Design review of the part shown in the three views and the two pictorial views. Dimensions are in mm from the part's minimum x, y and z. A direction names the side the tool comes from. Give positions to 0.01 mm unless a question says otherwise; leave off trailing zeros. Loops run counter-clockwise (first coordinate to the right, second up) from the corner with the lowest first, then second, coordinate; pieces in that order, holes last.
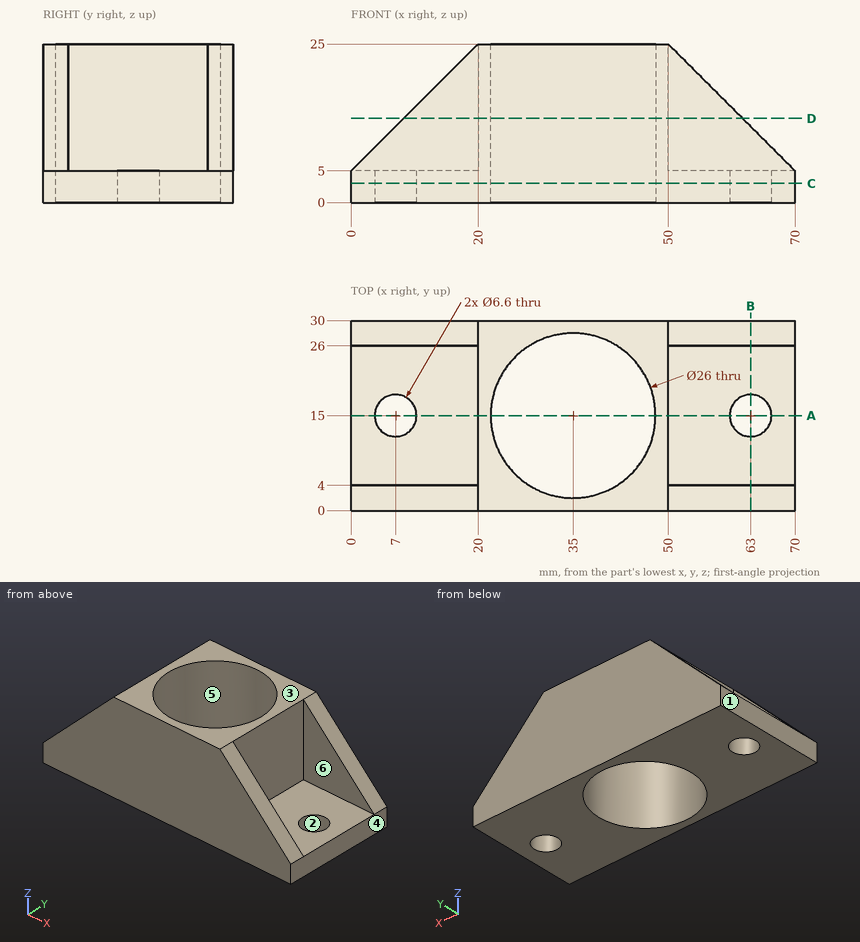
Q1. Wall thickness on line 1 (Y direction, x = 35, z = 15); line 2 (Y direction, x = 8.5, z = 7); line 3 (Z direction, x = 52, y = 22.25): over which ranges is each line inside the solid? List them lowest first.
Results:
line 1: y = 0 to 2, 28 to 30
line 2: y = 0 to 4, 26 to 30
line 3: z = 0 to 5
Q2. Take a section at D-D (z = 13.25). Give the boundary of the cut face in (x, y), plus the area to 3 significant figures.
Results:
outline: (8.25, 0) - (61.75, 0) - (61.75, 4) - (50, 4) - (50, 26) - (61.75, 26) - (61.75, 30) - (8.25, 30) - (8.25, 26) - (20, 26) - (20, 4) - (8.25, 4) - close; hole circle Ø26 at (35, 15)
area: 557 mm2
Q3. Take a section at A-A (y = 15). Give the boundary of the cut face in (x, z).
Results:
outline: (0, 0) - (3.7, 0) - (3.7, 5) - (0, 5) - close; (10.3, 0) - (22, 0) - (22, 25) - (20, 25) - (20, 5) - (10.3, 5) - close; (48, 0) - (59.7, 0) - (59.7, 5) - (50, 5) - (50, 25) - (48, 25) - close; (66.3, 0) - (70, 0) - (70, 5) - (66.3, 5) - close
Q4. Draft analysis for pull direction X (two halves, no side actions). For the marked faces 1, 2, 3 and 4, state which applies: pulls with the +X half, pulls with the -X half, needs draft (parallel to the pull), parting line crosses it, or undercut.
Results:
face 1: pulls with the -X half
face 2: undercut
face 3: needs draft
face 4: pulls with the +X half
Q5. Take a section at B-B (x = 63). Give the boundary of the cut face in (y, z).
Results:
outline: (0, 0) - (11.7, 0) - (11.7, 5) - (4, 5) - (4, 12) - (0, 12) - close; (18.3, 0) - (30, 0) - (30, 12) - (26, 12) - (26, 5) - (18.3, 5) - close
Q6. Take a section at C-C (z = 3). Give the boundary of the cut face in (x, y), plus the area to 3 significant figures.
Results:
outline: (0, 0) - (70, 0) - (70, 30) - (0, 30) - close; hole circle Ø6.6 at (7, 15); hole circle Ø26 at (35, 15); hole circle Ø6.6 at (63, 15)
area: 1,500 mm2
Q7. Tool access review of the marked faces 5 and 6: name each direction out of +Z, -Z, +X, -X, +Y, -Y from which nothing blocks a thin tool from reaching the whole face with its end or side.
Results:
face 5: +Z, -Z
face 6: +Z, +X
Q8. Insertion check: pin 1 (7.5 mm diameter, centred on x = 7, y = 15, fed in from -Z); pin 2 (8 mm diameter, centred on y = 7, z = 14.5, fed in from -X); pin 3 (6 mm diameter, centred on x = 13.5, y = 19, fed in from +Z); pin 4 (10 mm diameter, centred on y = 14.5, z = 15, fed in from -X). Each pin has a flat end and moves straight along its axis. Give the tip position at first contact, or say it passes through.
Results:
pin 1: stops at z = 0
pin 2: stops at x = 6.85
pin 3: stops at z = 5
pin 4: stops at x = 20
